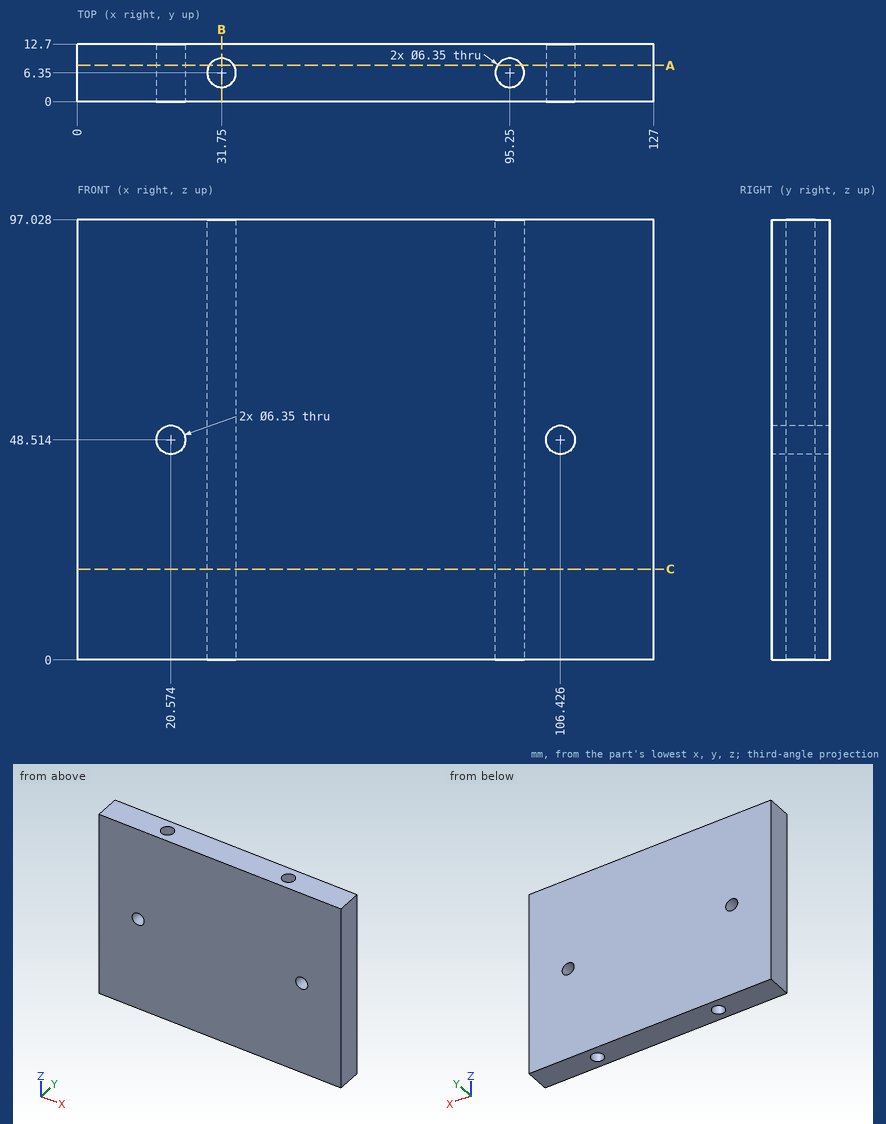
Input: dimensioned drawing with shaded views. Units: mm. Origin: part minimum x, y, z. Coordinates: 2 decimals unless noted, no trailing zeros. Write each loop counter-clockwise with the first axis right and the second up, starting at its lowest first coordinate (ties: lowest second). Pieces come first, ordered by that corner, then holes. Notation, with made-up numbers: M 46,-5.5 L 84,-5.5 A15 cw 84,21.5 Z; hole C 74,-18.5 d6. An arc over 180 degrees is marked long. Answer as CSV lines item,"result". Start each with the question number.
Q1. Cut plane C-C on z = 20. Return the cut outline in (x, y) (3 decimals).
Q2. Cut plane A-A on y = 8. Return the cut outline in (x, z) (3 decimals).
Q3. Cut plane B-B on x = 31.75. Return the cut outline in (y, z) (3 decimals).
Q4. Pin query (flat end, axial travel): P1, Ø4, axis at x = 106.426, z = 48.514, coming from the +Y side. Return the tip coordinate at first contact, or that it passes through.
Q5. Line query: line 1 (X direction, y = 6, z = 30); line 2 (Y direction, x = 31.75, z = 73) (3 decimals); line 3 (X direction, y = 11.5, z = 51). Output: solid intervals per line, ascending. Write a range as from..to.
Findings below:
1,outline,"M 0,0 L 127,0 L 127,12.7 L 0,12.7 Z; hole C 31.75,6.35 d6.35; hole C 95.25,6.35 d6.35"
2,outline,"M 0,0 L 29.037,0 L 29.037,97.028 L 0,97.028 Z; M 34.463,0 L 92.537,0 L 92.537,97.028 L 34.463,97.028 Z; M 97.963,0 L 127,0 L 127,97.028 L 97.963,97.028 Z; hole C 20.574,48.514 d6.35; hole C 106.426,48.514 d6.35"
3,outline,"M 0,0 L 3.175,0 L 3.175,97.028 L 0,97.028 Z; M 9.525,0 L 12.7,0 L 12.7,97.028 L 9.525,97.028 Z"
4,P1,"passes through"
5,line 1,"x = 0..28.59, 34.91..92.09, 98.41..127"
5,line 2,"y = 0..3.175, 9.525..12.7"
5,line 3,"x = 0..18.6, 22.55..104.45, 108.4..127"
